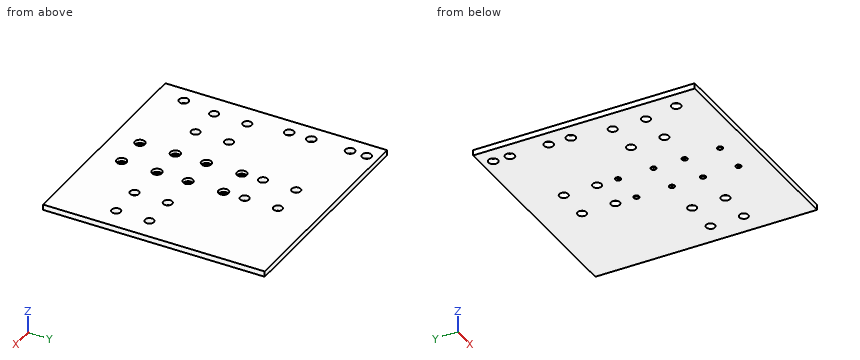
from build123d import *

# Parameters (mm, degrees)
F0_W     = 200
F0_H     = 5
F1_DEPTH = 200
F2_R     = 2.5
F3_DEPTH = 5.001
F4_R     = 4.25
F5_DEPTH = 5.001
F6_R     = 4.5
F7_DEPTH = 3
F8_R     = 4
F9_DEPTH = 25


with BuildPart() as f1:
    # F0 (on Right) → F1 (new body)
    with BuildSketch(Plane.YZ):
        with Locations((-100, 2.5)):
            Rectangle(F0_W, F0_H)
    extrude(amount=-F1_DEPTH)

    # F2 (on face) → F3 (cut, through all)
    with BuildSketch(Plane.XY.offset(5)):
        with Locations((-85, -84)):
            Circle(F2_R)
        with Locations((-115, -84)):
            Circle(F2_R)
        with Locations((-85, -116)):
            Circle(F2_R)
        with Locations((-115, -116)):
            Circle(F2_R)
        with Locations((-85, -144)):
            Circle(F2_R)
        with Locations((-115, -144)):
            Circle(F2_R)
        with Locations((-85, -176)):
            Circle(F2_R)
        with Locations((-115, -176)):
            Circle(F2_R)
    extrude(amount=-F3_DEPTH, mode=Mode.SUBTRACT)

    # F4 (on face) → F5 (cut, through all)
    with BuildSketch(Plane.XY.offset(5)):
        with Locations((-185, -25)):
            Circle(F4_R)
        with Locations((-185, -60)):
            Circle(F4_R)
        with Locations((-185, -10)):
            Circle(F4_R)
        with Locations((-185, -175)):
            Circle(F4_R)
        with Locations((-185, -80)):
            Circle(F4_R)
    extrude(amount=-F5_DEPTH, mode=Mode.SUBTRACT)

    # F6 (on face) → F7 (cut)
    with BuildSketch(Plane.XY.offset(5)):
        with Locations((-115, -84)):
            Circle(F6_R)
        with Locations((-85, -84)):
            Circle(F6_R)
        with Locations((-115, -116)):
            Circle(F6_R)
        with Locations((-85, -116)):
            Circle(F6_R)
        with Locations((-115, -144)):
            Circle(F6_R)
        with Locations((-85, -144)):
            Circle(F6_R)
        with Locations((-115, -176)):
            Circle(F6_R)
        with Locations((-85, -176)):
            Circle(F6_R)
    extrude(amount=-F7_DEPTH, mode=Mode.SUBTRACT)

    # F8 (on face) → F9 (cut)
    with BuildSketch(Plane.XY.offset(5)):
        with Locations((-150, -145)):
            Circle(F8_R)
        with Locations((-180, -145)):
            Circle(F8_R)
        with Locations((-20, -145)):
            Circle(F8_R)
        with Locations((-50, -145)):
            Circle(F8_R)
        with Locations((-20, -115)):
            Circle(F8_R)
        with Locations((-50, -115)):
            Circle(F8_R)
        with Locations((-150, -115)):
            Circle(F8_R)
        with Locations((-180, -115)):
            Circle(F8_R)
        with Locations((-85, -65)):
            Circle(F8_R)
        with Locations((-85, -35)):
            Circle(F8_R)
        with Locations((-115, -35)):
            Circle(F8_R)
        with Locations((-115, -65)):
            Circle(F8_R)
    extrude(amount=-F9_DEPTH, mode=Mode.SUBTRACT)


solid = f1.part
Here's how the part is built. I have some questions about the finished solid (model axes, mm). Round coordinates to 2 decimals unless told otherwise and drop trailing zeros. Order: outer loops, then holes, each group sorted by start corner. A loop starts at its lowest first (then second) coordinate and runs counter-clockwise, first axis right, second up. Notation, with made-up numbers: (29.5, -19) -> (64.5, -19) arc R23 ccw to (64.5, -11) -> close; hole circle Ø11 at (63.5, 28). An arc over 180 degrees is marked (long way). Use CSV: the item, a comma, the result in double quotes.
1. I'm going to push flat-ended pins straight in: P1, Ø6, axis at x = -115, y = -144, coming from the +Z side; P2, Ø5, axis at x = -50, y = -145, coming from the -Z side. Where does each tip first touch, or does it pass through?
Recorded:
P1,"stops at z = 2"
P2,"passes through"
2. I need wall thicknesses on line 1 along X through (y, z) = (-34.5, 2.25); line 2 along Y through (x, z) = (-150, 3.05); line 3 along Y through (x, z) = (-177, 1.2). Which ranges of each line are inside material? Lowest first, please.
Recorded:
line 1,"x = -200 to -118.97, -111.03 to -88.97, -81.03 to 0"
line 2,"y = -200 to -149, -141 to -119, -111 to 0"
line 3,"y = -200 to -147.65, -142.35 to -117.65, -112.35 to 0"
3. I want a section at B-B on y = -10. List the corners of the cut face in (x, z) for me.
Recorded:
outline,"(-200, 0) -> (-189.25, 0) -> (-189.25, 5) -> (-200, 5) -> close; (-180.75, 0) -> (0, 0) -> (0, 5) -> (-180.75, 5) -> close"
4. I want a section at A-A on y = -35. List the corners of the cut face in (x, z) for me, and give its area (3 significant figures).
Recorded:
outline,"(-200, 0) -> (-119, 0) -> (-119, 5) -> (-200, 5) -> close; (-111, 0) -> (-89, 0) -> (-89, 5) -> (-111, 5) -> close; (-81, 0) -> (0, 0) -> (0, 5) -> (-81, 5) -> close"
area,"920 mm2"
5. I want a section at D-D on x = -151.5. List the corners of the cut face in (y, z) for me.
Recorded:
outline,"(-200, 0) -> (-148.71, 0) -> (-148.71, 5) -> (-200, 5) -> close; (-141.29, 0) -> (-118.71, 0) -> (-118.71, 5) -> (-141.29, 5) -> close; (-111.29, 0) -> (0, 0) -> (0, 5) -> (-111.29, 5) -> close"
6. I want a section at C-C on z = 1.25. Give the number of separate pieces and of enclosed holes in the cut face, and give its area (3 significant figures).
Recorded:
separate pieces,"1"
enclosed holes,"25"
area,"39,000 mm2"
